Source: CAD feature listing. Evaluate the final solid. Frame: model axes, mm. Give positions to 0.01 mm unless a question says otherwise; leave off trailing zeros. Loops run counter-clockwise (first coordinate to the right, second up) from the corner with the lowest first, then second, coordinate; pieces in that order, holes last. Notation, with made-up numbers: (69, 39) - (124, 39) arc R18 ccw to (124, 61) - close; hole circle Ø1 at (-35.5, -40). An arc over 180 degrees is marked (long way). Put each result on its own line as item: value.
```python
from build123d import *

# Parameters (mm, degrees)
BOSS_EXTRUDE1_DEPTH = 10
FILLET1_R           = 3
SKETCH2_R           = 1
CUT_EXTRUDE1_DEPTH  = 130.65


with BuildPart() as part:
    # Sketch1 → Boss-Extrude1 (new body)
    with BuildSketch(Plane(origin=(0, 0, 0), x_dir=(1, 0, 0), z_dir=(0, 1, 0))):
        Polygon((0, 0), (0, -34.15), (-130.65, -34.15), (-130.65, 0), (-130.5, 0), (-130.5, -34), (-0.15, -34), (-0.15, 0), align=None)
    extrude(amount=BOSS_EXTRUDE1_DEPTH)

    # Fillet1
    fillet1_edges = [part.edges().sort_by_distance(p)[0] for p in [
        (-0.075, 10, 0),
        (-130.575, 10, 0),
        (-130.575, 0, 0),
        (-0.075, 0, 0),
    ]]
    fillet(fillet1_edges, radius=FILLET1_R)

    # Sketch2 → Cut-Extrude1 (cut)
    with BuildSketch(Plane(origin=(0, 0, 0), x_dir=(0, 0, -1), z_dir=(1, 0, 0))):
        with Locations((-6.25, 5)):
            Circle(SKETCH2_R)
        with Locations((-24.75, 5)):
            Circle(SKETCH2_R)
    extrude(amount=-CUT_EXTRUDE1_DEPTH, mode=Mode.SUBTRACT)


solid = part.part
```
1) Mould query, pull axis X, two halves, no side actions, for faces 1 (the flat face through (-130.5, 5, 17)), 2 (the flat face through (-130.65, 5, 17)). Classes: pulls with the +X half, pulls with the -X half, needs draft (parallel to the pull), parting line crosses it, or undercut.
Check result:
face 1: undercut
face 2: pulls with the -X half
2) Material intervals for line 1 along X through (y, z) = (9.25, 13); line 2 along Y through (x, z) = (-130.6, 6.25), sorted ascending. Write a range as [from, to].
Check result:
line 1: [-130.65, -130.5], [-0.15, 0]
line 2: [0, 4], [6, 10]
3) Pin query (flat end, axial travel): P1, Ø5, axis at x = -90.5, y = 6.5, coming from the -Z side; P2, Ø3, axis at y = 5, z = 6.25, coming from the +X side. Return the tip coordinate at first contact, or that it passes through.
Check result:
P1: z = 34
P2: x = 0
4) Section query A-A, the plane z = 20.5. Output: boundary loops of the cut face in (x, y), plus the area to 3 significant figures.
Check result:
outline: (-130.65, 0) - (-130.5, 0) - (-130.5, 10) - (-130.65, 10) - close; (-0.15, 0) - (0, 0) - (0, 10) - (-0.15, 10) - close
area: 3.00 mm²
5) Section query B-B, the plane y = 8.5. Output: boundary loops of the cut face in (x, z), plus the area to 3 significant figures.
Check result:
outline: (-130.65, 0.4) - (-130.5, 0.4) - (-130.5, 34) - (-0.15, 34) - (-0.15, 0.4) - (0, 0.4) - (0, 34.15) - (-130.65, 34.15) - close
area: 29.7 mm²
6) Section query C-C, the plane x = -106. Output: boundary loops of the cut face in (y, z), plus the area to 3 significant figures.
Check result:
outline: (0, 34) - (10, 34) - (10, 34.15) - (0, 34.15) - close
area: 1.50 mm²
